The drawing under review shows one solid part. Ordinate dimensions are in mm from its lowest x, y, z. A direction names the side the tool comes from. Give positions to 0.01 mm unless a question says otherwise; leave off trailing zeros. Order: outer loops, then holes, each group sorted by start corner. A loop starts at its lowest first (then second) coordinate and runs counter-clockwise, first axis right, second up. Notation, with made-up numbers: (13, -30) - (41, -30) arc R31 cw to (41, 5) - close; hole circle Ø6 at (49.5, 15). An arc over 180 degrees is marked (long way). Use CSV: the item, a comma, the result in double quotes. Start each with the question number.
1. Machinability: for the marked faces 1, 2 and 3, which of the approach directions +Z, -Z, +X, -X, +Y, -Y give a long, thin tool a straight path to every point of the face, cutting with its end or side? Answer none if there is none.
2. Take a section at B-B, the plane y = 48.5. State the section outline as (x, z) points, then the cut area to 3 significant figures.
3. Draft analysis for pull direction Z (two halves, no side actions). For the marked faces 4, 5 and 6, state which applies: released by +Z, released by -Z, zero draft, split by the parting line, or undercut.
4. Take a section at A-A, the plane z = 18.5. State the section outline as (x, y) points (1 decimal).
5. Take a section at C-C, the plane x = 3.5. Count the separate pieces of the cut face and the enclosed holes in it, then the cut area to 3 significant figures.
6. To check wall thickness, follow line 1 (X direction, y = 45, z = 51); line 2 (Z direction, x = 6, y = 23.5) (1 decimal); line 3 (Z direction, x = 2, y = 33) (1 decimal). State the ranges of each line that lie inside material, in increasing order. Write a range as [from, to].
7. For pin 1 (6 mm diameter, centred on x = 16.5, y = 29.5, fed in from -Z); pin 2 (5 mm diameter, centred on x = 16, z = 42, fed in from +Y); pin 3 (1 mm diameter, centred on y = 26.5, z = 45.5, fed in from +X), all flat-tipped, find the tip position at first contact; note any pin that passes through.
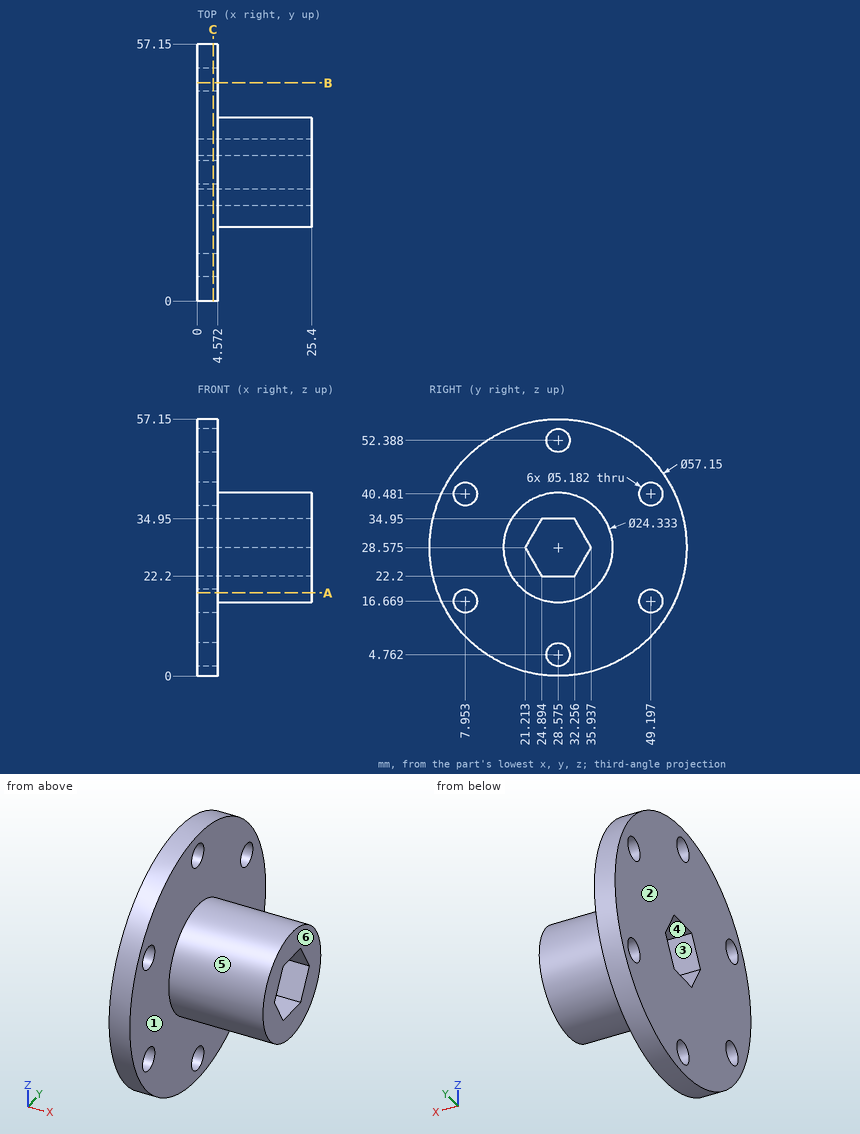
Determined:
1,face 1,"+X"
1,face 2,"+Z, -Z, -X, +Y, -Y"
1,face 3,"+X, -X"
2,outline,"(0, 8.09) - (4.57, 8.09) - (4.57, 14.17) - (0, 14.17) - close; (0, 19.16) - (4.57, 19.16) - (4.57, 37.99) - (0, 37.99) - close; (0, 42.98) - (4.57, 42.98) - (4.57, 49.06) - (0, 49.06) - close"
2,area,"142 mm²"
3,face 4,"undercut"
3,face 5,"split by the parting line"
3,face 6,"zero draft"
4,outline,"(0, 1.8) - (4.6, 1.8) - (4.6, 6.1) - (0, 6.1) - close; (0, 9.8) - (4.6, 9.8) - (4.6, 21.8) - (25.4, 21.8) - (25.4, 35.4) - (4.6, 35.4) - (4.6, 47.4) - (0, 47.4) - close; (0, 51) - (4.6, 51) - (4.6, 55.3) - (0, 55.3) - close"
5,separate pieces,"1"
5,enclosed holes,"7"
5,area,"2,300 mm²"
6,line 1,"x = [0, 4.57]"
6,line 2,"z = [17.5, 24.6], [32.5, 39.6]"
6,line 3,"z = [0.3, 23.5], [33.7, 56.8]"
7,pin 1,"stops at z = 16.41"
7,pin 2,"stops at y = 33.93"
7,pin 3,"stops at x = 4.57"
